The model under review builds one solid part; all positions refer to its coordinate system, in mm. A direction names the side the tool comes from. Coordinates: 2 decimals unless noted, no trailing zeros. Order: outer loops, then holes, each group sorted by start corner. A loop starts at its lowest first (then second) coordinate and runs counter-clockwise, first axis right, second up. Notation, with made-up numbers: (-32, -35) -> (-10, -35) arc R32 ccw to (-10, -8) -> close; hole circle Ø11 at (3, 86). An arc over 180 degrees is marked (long way). Use one line per item in the form item = value. Start each with the question number.
(1) Take a section at B-B (y = -2). State the section outline as (x, z) points (1 decimal).
(2) Wall thickness on line 1 along X through (y, z) = (-1.6, -3.5); line 2 along X through (y, z) = (-1.5, -3.5); line 3 along Y through (x, z) = (5, -7.25): over which ranges is each line inside the solid? List them lowest first.
(3) For faces 1 (the cylindrical face through (6.38, 6.8, -7.67)), 2 (the cylindrical face through (0, -8, -3)), 3 (the flat face through (11, 0.5, -8)), 4 (the flat face through (9.5, 5, -3)), list the 3-axis set-ups (+Z, -Z, +X, -X, +Y, -Y) from which the entire face can be reached by the end or side of a thin tool; tool diameter is ignored.
(4) Mouldability with a two-part tool opening along Y and no side actions: class faces 5 (the flat face through (15.5, 2, -6)), 6 (the cylindrical face through (11.65, -4.828, -6.261)), 7 (the cylindrical face through (10.93, 4.606, -6.679)) as +Y half, -Y half, draft (parallel to the pull), parting line (faces both ways), or undercut.
(5) Take a section at A-A (x = 0). State the section outline as (y, z) points, then the cut area to 3 significant figures.
(6) Take a section at C-C (z = -4.5). State the section outline as (x, y) points (1 decimal).
(7) Take a section at D-D (x = 13). State the section outline as (y, z) points.
(8) Insertion check: pin 1 Ø6.5 at (x, z) = (12, -3.5) entering from +Y; pin 2 Ø5 at (x, z) = (12, -5.5) entering from -Y; pin 3 Ø4.5 at (x, y) = (5.66, -5.66) entering from -Z; pin 4 Ø3.5 at (x, z) = (13, -3.5) entering from -Y. Each pin has a flat end and moves straight along its axis. Give the tip position at first contact, or say it passes through.
```python
from build123d import *

# Parameters (mm, degrees)
CUT_EXTRUDE1_START     = -12.7
CUT_EXTRUDE1_DEPTH     = 12.7
CUT_EXTRUDE1_START_2   = -7.233059634
CUT_EXTRUDE1_2_DEPTH   = 7.233059634
CUT_EXTRUDE1_3_DEPTH   = 6
CUT_EXTRUDE1_4_DEPTH   = 1.533059634
CUT_EXTRUDE1_START_3   = 9.5
CUT_EXTRUDE1_5_DEPTH   = 6.5
SKETCH3_W              = 1.3525
SKETCH3_H              = 10.6
M2_5_CLEARANCE_HOLE2_D = 2.705
SKETCH7_W              = 1.85
SKETCH7_H              = 10.6


with BuildPart() as part:
    # Cut-Extrude1: read off the stored shape, not the designer's step
    # Cut-Extrude1 outline → Cut-Extrude1 (new body)
    with BuildSketch(Plane(origin=(0, 0, -12.7), x_dir=(-1, 0, 0), z_dir=(0, 0, -1)).offset(CUT_EXTRUDE1_START)):
        with BuildLine():
            Line((-5.678027827, -0.5), (-15.5, -0.5))
            Line((-15.5, -0.5), (-15.5, -4))
            ThreePointArc((-15.5, -4), (-11.598248501, -4.851105882), (-8.405387738, -7.249790133))
            ThreePointArc((-8.405387738, -7.249790133), (11.1, 0), (-8.405387738, 7.249790133))
            ThreePointArc((-8.405387738, 7.249790133), (-8.930606577, 6.689081827), (-9.5, 6.173291403))
            Line((-9.5, 6.173291403), (-9.5, 4))
            Line((-9.5, 4), (-15.5, 4))
            Line((-15.5, 4), (-15.5, 0.5))
            Line((-15.5, 0.5), (-5.678027827, 0.5))
            ThreePointArc((-5.678027827, 0.5), (-5.7, 0), (-5.678027827, -0.5))
        make_face()
    extrude(amount=CUT_EXTRUDE1_DEPTH)

    # Cut-Extrude1 2 outline → Cut-Extrude1 2 (add)
    with BuildSketch(Plane(origin=(0, 0, -12.7), x_dir=(-1, 0, 0), z_dir=(0, 0, -1)).offset(CUT_EXTRUDE1_START_2)):
        with BuildLine():
            ThreePointArc((-9.5, 6.173291403), (-12.309263583, 4.560062613), (-15.5, 4))
            Line((-15.5, 4), (-9.5, 4))
            Line((-9.5, 4), (-9.5, 6.173291403))
        make_face()
    extrude(amount=CUT_EXTRUDE1_2_DEPTH)

    # Cut-Extrude1 3 outline → Cut-Extrude1 3 (add)
    with BuildSketch(Plane(origin=(0, 0, -12.7), x_dir=(-1, 0, 0), z_dir=(0, 0, -1)).offset(CUT_EXTRUDE1_START)):
        with BuildLine():
            ThreePointArc((-7.984359711, 0.5), (-8, 0), (-7.984359711, -0.5))
            Line((-7.984359711, -0.5), (-5.678027827, -0.5))
            ThreePointArc((-5.678027827, -0.5), (-5.7, 0), (-5.678027827, 0.5))
            Line((-5.678027827, 0.5), (-7.984359711, 0.5))
        make_face()
    extrude(amount=CUT_EXTRUDE1_3_DEPTH)

    # Cut-Extrude1 4 outline → Cut-Extrude1 4 (add)
    with BuildSketch(Plane(origin=(0, 0, -12.7), x_dir=(-1, 0, 0), z_dir=(0, 0, -1)).offset(CUT_EXTRUDE1_START)):
        with BuildLine():
            ThreePointArc((-9.5, 6.173291403), (-12.309263583, 4.560062613), (-15.5, 4))
            Line((-15.5, 4), (-9.5, 4))
            Line((-9.5, 4), (-9.5, 6.173291403))
        make_face()
    extrude(amount=CUT_EXTRUDE1_4_DEPTH)

    # Cut-Extrude1 5 outline → Cut-Extrude1 5 (cut)
    with BuildSketch(Plane.YZ.offset(CUT_EXTRUDE1_START_3)):
        with BuildLine():
            ThreePointArc((6.173291403, -1.533059534), (5.2222696, -0.629576076), (4, -0.153359894))
            Line((4, -0.153359894), (4, -1.533059634))
            Line((4, -1.533059634), (6.173291403, -1.533059534))
        make_face()
        with BuildLine():
            Line((6.173291403, -5.466940466), (4, -5.466940366))
            Line((4, -5.466940366), (4, -6.846640106))
            ThreePointArc((4, -6.846640106), (5.2222696, -6.370423924), (6.173291403, -5.466940466))
        make_face()
    extrude(amount=CUT_EXTRUDE1_5_DEPTH, mode=Mode.SUBTRACT)

    # Sketch2 → Cut-Revolve1 (revolve, cut)
    with BuildSketch(Plane(origin=(0, 0, 0), x_dir=(1, 0, 0), z_dir=(0, 1, 0))):
        Polygon((5.7, 12.7), (0, 12.7), (0, 0), (8, 0), (8, 6), (5.7, 6), align=None)
    revolve(axis=Axis((0, 0, -12.7), (0, 0, 1)), mode=Mode.SUBTRACT)

    # Sketch3 → M2.5 Clearance Hole1 (revolve, cut)
    with BuildSketch(Plane(origin=(13, -0.5, -3.5), x_dir=(0, 0, 1), z_dir=(1, 0, 0))):
        with Locations((0.67625, 5.3)):
            Rectangle(SKETCH3_W, SKETCH3_H)
    revolve(axis=Axis((13, 5.85, -3.5), (0, -1, 0)), mode=Mode.SUBTRACT)

    # M2.5 Clearance Hole2 (through all)
    with Locations(Plane(origin=(0, 0, -12.7), x_dir=(-1, 0, 0), z_dir=(0, 0, -1))):
        with Locations((-5.656854249, -5.656854249), (5.656854249, -5.656854249), (5.656854249, 5.656854249), (-5.656854249, 5.656854249)):
            Hole(M2_5_CLEARANCE_HOLE2_D / 2)

    # Sketch7 → Ø3.7 (3.7) Diameter Hole1 (revolve, cut)
    with BuildSketch(Plane(origin=(13, 0.5, -3.5), x_dir=(0, 0, -1), z_dir=(1, 0, 0))):
        with Locations((0.925, 5.3)):
            Rectangle(SKETCH7_W, SKETCH7_H)
    revolve(axis=Axis((13, -5.85, -3.5), (0, 1, 0)), mode=Mode.SUBTRACT)


solid = part.part
```
Findings:
q1.outline = (-10.9, -12.7) -> (-5.3, -12.7) -> (-5.3, -6) -> (-7.7, -6) -> (-7.7, 0) -> (-10.9, 0) -> close; (5.3, -12.7) -> (15.5, -12.7) -> (15.5, 0) -> (7.7, 0) -> (7.7, -6) -> (5.3, -6) -> close; hole circle Ø2.7 at (13, -3.5)
q2.line_1 = -10.98 to -7.84, 7.84 to 11.65, 14.35 to 15.5
q2.line_2 = -11 to -7.86, 7.86 to 11.65, 14.35 to 15.5
q2.line_3 = -9.91 to -6.84, -4.47 to -2.74, 2.74 to 4.47, 6.84 to 9.91
q3.face_1 = +Z, -Z
q3.face_2 = +Z
q3.face_3 = +Z, -Z, +X
q3.face_4 = +X
q4.face_5 = draft
q4.face_6 = -Y half
q4.face_7 = undercut
q5.outline = (-11.1, -12.7) -> (-5.7, -12.7) -> (-5.7, -6) -> (-8, -6) -> (-8, 0) -> (-11.1, 0) -> close; (5.7, -12.7) -> (11.1, -12.7) -> (11.1, 0) -> (8, 0) -> (8, -6) -> (5.7, -6) -> close
q5.area = 110 mm²
q6.outline = (-6.5, -4.6) arc R8 cw to (-6.5, 4.6) arc R1.4 cw (long way) to (-4.6, 6.5) arc R8 cw to (4.6, 6.5) arc R1.4 cw (long way) to (6.5, 4.6) arc R8 cw to (8, 0.5) -> (11.4, 0.5) -> (11.4, 4) -> (9.5, 4) -> (9.5, 6.2) arc R9.4 cw to (8.4, 7.2) arc R11.1 ccw (long way) to (8.4, -7.2) arc R9.4 cw to (12.1, -4.6) -> (12.1, -0.5) -> (8, -0.5) arc R8 cw to (6.5, -4.6) arc R1.4 cw (long way) to (4.6, -6.5) arc R8 cw to (-4.6, -6.5) arc R1.4 cw (long way) to start; (13.9, -4.1) arc R9.4 cw to (15.5, -4) -> (15.5, -0.5) -> (13.9, -0.5) -> close; (14.6, 0.5) -> (15.5, 0.5) -> (15.5, 4) -> (14.6, 4) -> close
q7.outline = (-4.34, -12.7) -> (-0.5, -12.7) -> (-0.5, -4.85) -> (-4.34, -4.85) -> close; (-4.34, -2.15) -> (-0.5, -2.15) -> (-0.5, 0) -> (-4.34, 0) -> close; (0.5, -12.7) -> (4.34, -12.7) -> (4.34, -6.77) arc R3.4 cw to (4, -6.85) -> (4, -5.35) -> (0.5, -5.35) -> close; (0.5, -1.65) -> (4, -1.65) -> (4, -0.15) arc R3.4 cw to (4.34, -0.23) -> (4.34, 0) -> (0.5, 0) -> close
q8.pin_1 = 6.87
q8.pin_2 = -6.17
q8.pin_3 = -12.7
q8.pin_4 = -5.02
